Source: CAD feature listing. Evaluate the final solid. Frame: model axes, mm. A direction names the side the tool comes from. Round coordinates to 2 decimals unless told otherwise and drop trailing zeros. Loops run counter-clockwise (first coordinate to the right, second up) from the corner with the lowest first, then second, coordinate; pieces in that order, holes last.
(1) Section B-B, the plane x = -11.25. Return the cut outline in (y, z), plus the area to 3 significant figures.
(2) Section D-D, the plane y = 16.5. Return the cut outline in (x, z).
(3) Material intervals for probe 1 along X at (y, z) = (0, 6.9); probe 2 along Y at (x, z) = (-11.25, 7.7); probe 3 along Y at (x, z) = (12, 8.25), sorted ascending.
(4) Set-up query: faces 1 (the cylindrical face through (7.46, -13.48, 7.08)), 2 (the flat face through (0, -18, 5)), 3 (the flat face through (-9, 0, 0.5)). Return all of +Z, -Z, +X, -X, +Y, -Y with unobstructed straight access to the full face (end or side cutting, diameter ignored); none if empty.
(5) Mould query, pull axis X, two halves, no side actions, for faces 4 (the flat face through (-15.25, 0, 4)), 5 (the flat face through (0, 0, 8.35)), 6 (the cylindrical face through (8.8, -10.93, 2.88)), 7 (the cylindrical face through (8.8, 13.07, 2.88)). Classes: pulls with the +X half, pulls with the -X half, needs draft (parallel to the pull), parting line crosses it, or undercut.
(6) Section A-A, the plane z = 2.75. Return the cut outline in (x, y), plus the area to 3 significant figures.
(7) Section C-C, the plane y = -12. Return the cut outline in (x, z), plus the area to 3 significant figures.
(8) First-contact query: pin 1 Ø4.5 at (x, y) = (9, -11.5) entering from +Z; pin 2 Ø4.5 at (x, y) = (-11.25, 0) entering from -Z; pin 3 Ø4.5 at (x, y) = (9.78, 0) entering from +Z. Flat tips, straight axial feed; report the tip coordinate or a pass-through.
Autodesk Inventor part; units mm, degrees
ref_plane "YZ Plane" through (0, 0, 0) normal (1, 0, 0) x (0, 1, 0)
ref_plane "XZ Plane" through (0, 0, 0) normal (0, 1, 0) x (-1, 0, 0)
ref_plane "XY Plane" through (0, 0, 0) normal (0, 0, 1) x (1, 0, 0)
sketch "Sketch1" plane through (0, 0, 0) normal (0, 0, 1) x (1, 0, 0)
  line L0 (-15.25, 18) -> (15.25, 18)
  line L1 (15.25, 18) -> (15.25, -18)
  line L2 (15.25, -18) -> (-15.25, -18)
  line L3 (-15.25, -18) -> (-15.25, 18)
  point P0 (0, 0)
  dimension "d0" = 30.5
  dimension "d1" = 36
  dimension "d2" = 18
  dimension "d3" = 15.25
extrude "Extrusion1" add sketch "Sketch1" along normal blind 8.35
sketch "Sketch2" plane through (-15.25, 18, 0) normal (0, 1, 0) x (1, 0, 0)
  line L0 (30.5, 0) -> (30.5, -8.35)
  line L1 (30.5, -8.35) -> (70.5, -8.35)
  line L2 (70.5, 11.65) -> (70.5, -8.35)
  line L3 (0, 11.65) -> (70.5, 11.65)
  line L4 (0, 11.65) -> (0, 0.5)
  line L5 (0, 0.5) -> (9.7766, 0.5)
  arc A0 (19.2498, 0) -> (9.7766, 0.5) centre (14.5, 0) ccw
  line L6 (19.2498, 0) -> (30.5, 0)
  circle A1 centre (40.5, 1.65) radius 0.847
  circle A2 centre (62.5, 1.65) radius 0.847
  circle A3 centre (54.5, 1.65) radius 4
  circle A4 centre (14.5, 0) radius 4.7498
  point P0 (15.25, 0)
extrude "Extrusion2" cut sketch "Sketch2" against normal through all contours A4 A0
sketch "Sketch3" plane through (0, 0, 8.35) normal (0, 0, 1) x (1, 0, 0)
  circle A0 centre (-11.25, 12) radius 1.0065
  circle A1 centre (-11.25, 0) radius 1.0065
  circle A2 centre (-11.25, -12) radius 1.0065
  circle A3 centre (9.7764, 12) radius 1.0065
  circle A4 centre (9.7764, 0) radius 1.0065
  circle A5 centre (9.7764, -12) radius 1.0065
  point P0 (0, 0)
hole "CBore for M2.5 screw" at (-11.25, -12, 8.35) at (-11.25, 0, 8.35) at (-11.25, 12, 8.35) at (9.7764, -12, 8.35) at (9.7764, 0, 8.35) at (9.7764, 12, 8.35) direction (0, 0, -1) diameter 2.9 end through all counterbore diameter 5.5 counterbore depth 2.5
sketch "Sketch4" plane through (0, 0, 0) normal (0, 0, -1) x (-1, 0, 0)
  circle A0 centre (11.25, 0) radius 1.45
  circle A1 centre (11.25, -12) radius 1.45
  circle A2 centre (11.25, 12) radius 1.45
  line L0 (5.4998, 18) -> (5.4998, -18)
  line L1 (5.4998, -18) -> (15.25, -18)
  line L2 (15.25, -18) -> (15.25, 18)
  line L3 (15.25, 18) -> (5.4998, 18)
  line L4 (15.25, -18) -> (4.4998, -18)
  line L5 (4.4998, -18) -> (4.4998, 18)
  line L6 (4.4998, 18) -> (15.25, 18)
  line L7 (15.25, 18) -> (15.25, -18)
  point P0 (0, 0)
  dimension "d17" = 1
extrude "Extrusion3" cut sketch "Sketch4" against normal blind 0.5
properties part number "J007580" material "ALUMINUM, 6061-T651"
Output values:
1. outline: (-18, 0.5) - (-13.45, 0.5) - (-13.45, 5.85) - (-14.75, 5.85) - (-14.75, 8.35) - (-18, 8.35) - close; (-10.55, 0.5) - (-1.45, 0.5) - (-1.45, 5.85) - (-2.75, 5.85) - (-2.75, 8.35) - (-9.25, 8.35) - (-9.25, 5.85) - (-10.55, 5.85) - close; (1.45, 0.5) - (10.55, 0.5) - (10.55, 5.85) - (9.25, 5.85) - (9.25, 8.35) - (2.75, 8.35) - (2.75, 5.85) - (1.45, 5.85) - close; (13.45, 0.5) - (18, 0.5) - (18, 8.35) - (14.75, 8.35) - (14.75, 5.85) - (13.45, 5.85) - close
1. area: 195 mm2
2. outline: (-15.25, 0.5) - (-5.47, 0.5) arc R4.75 cw to (4, 0) - (15.25, 0) - (15.25, 8.35) - (-15.25, 8.35) - close
3. probe 1: x = -15.25 to -14, -8.5 to 7.03, 12.53 to 15.25
3. probe 2: y = -18 to -14.75, -9.25 to -2.75, 2.75 to 9.25, 14.75 to 18
3. probe 3: y = -18 to -13.62, -10.38 to -1.62, 1.62 to 10.38, 13.62 to 18
4. face 1: +Z
4. face 2: +Z, -Z, +X, -X, -Y
4. face 3: -Z, -X, +Y, -Y
5. face 4: pulls with the -X half
5. face 5: needs draft
5. face 6: undercut
5. face 7: undercut
6. outline: (-15.25, -18) - (-4.62, -18) - (-4.62, 18) - (-15.25, 18) - close; (3.12, -18) - (15.25, -18) - (15.25, 18) - (3.12, 18) - close; hole circle Ø2.9 at (-11.25, -12); hole circle Ø2.9 at (-11.25, 0); hole circle Ø2.9 at (-11.25, 12); hole circle Ø2.9 at (9.78, -12); hole circle Ø2.9 at (9.78, 0); hole circle Ø2.9 at (9.78, 12)
6. area: 780 mm2
7. outline: (-15.25, 0.5) - (-12.7, 0.5) - (-12.7, 5.85) - (-14, 5.85) - (-14, 8.35) - (-15.25, 8.35) - close; (-9.8, 0.5) - (-5.47, 0.5) arc R4.75 cw to (4, 0) - (8.33, 0) - (8.33, 5.85) - (7.03, 5.85) - (7.03, 8.35) - (-8.5, 8.35) - (-8.5, 5.85) - (-9.8, 5.85) - close; (11.23, 0) - (15.25, 0) - (15.25, 8.35) - (12.53, 8.35) - (12.53, 5.85) - (11.23, 5.85) - close
7. area: 154 mm2
8. pin 1: stops at z = 8.35
8. pin 2: stops at z = 0.5
8. pin 3: stops at z = 5.85
